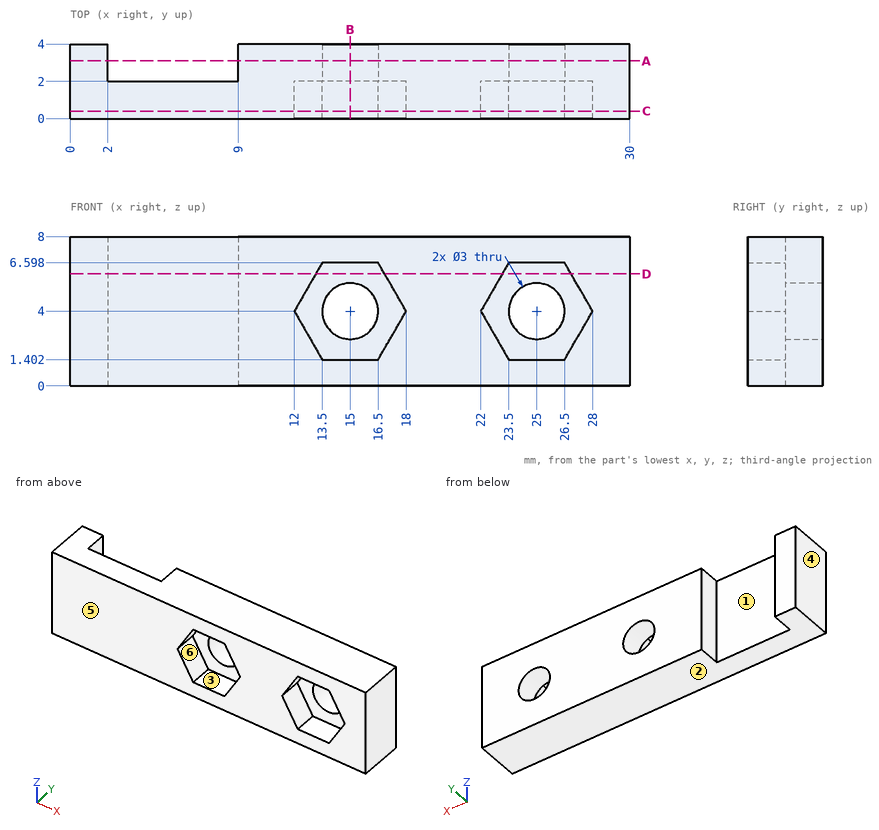
Verification items for this drawing (mm, ordinates from the low corner). A direction names the side the tool comes from. Round coordinates to 2 decimals unless told otherwise and drop trailing zeros. Loops run counter-clockwise (first coordinate to the right, second up) from the corner with the lowest first, then second, coordinate; pieces in that order, holes last. Notation, with made-up numbers: (79, 1.5) -> (107, 1.5) arc R21 ccw to (107, 17.5) -> close; hole circle Ø10 at (3, 49.25). An arc over 180 degrees is marked (long way). Write item = value, one per line. Start each with the question number.
1) Sectioned sample at C-C, the plane y = 0.4. Record the cut outline in (x, z).
2) Thickness scan on probe 1 along X at (y, z) = (3.1, 4); probe 2 along Z at (x, y) = (15.5, 1.3); probe 3 along X at (y, z) = (0.75, 2) (1 decimal). Record the ranges inside material, lowest first.
3) Sectioned sample at D-D, the plane z = 6. Record the cut outline in (x, y).
4) Gauge pin test, flat ends, axial feed: pin 1 Ø1.5 at (x, z) = (16, 5) entering from +Y; pin 2 Ø2.5 at (x, z) = (15, 3.5) entering from -Y; pin 3 Ø4 at (x, z) = (5, 2) entering from +Y. Record the tip position at first contact, or that the pin passes through.
5) Sectioned sample at A-A, the plane y = 3.1. Record the cut outline in (x, z), plus the area to 3 significant figures.
6) Release check for a two-part mould opening along X. For the marked faces 4, 5 and 6 record: released by +X, released by -X, zero draft, split by the parting line, or undercut.
7) Sectioned sample at B-B, the plane x = 15. Record the cut outline in (y, z).
8) Set-up check for the marked faces 1, 2 and 3: record each of +Z, -Z, +X, -X, +Y, -Y from which the full face is reachable in a straight line by a thin tool's end or side.
Results are:
q1.outline = (0, 0) -> (30, 0) -> (30, 8) -> (0, 8) -> close; hole (12, 4) -> (13.5, 1.4) -> (16.5, 1.4) -> (18, 4) -> (16.5, 6.6) -> (13.5, 6.6) -> close; hole (22, 4) -> (23.5, 1.4) -> (26.5, 1.4) -> (28, 4) -> (26.5, 6.6) -> (23.5, 6.6) -> close
q2.probe_1 = 0 to 2, 9 to 13.5, 16.5 to 23.5, 26.5 to 30
q2.probe_2 = 0 to 1.4, 6.6 to 8
q2.probe_3 = 0 to 13.2, 16.8 to 23.2, 26.8 to 30
q3.outline = (0, 0) -> (13.15, 0) -> (13.15, 2) -> (16.85, 2) -> (16.85, 0) -> (23.15, 0) -> (23.15, 2) -> (26.85, 2) -> (26.85, 0) -> (30, 0) -> (30, 4) -> (9, 4) -> (9, 2) -> (2, 2) -> (2, 4) -> (0, 4) -> close
q4.pin_1 = 4
q4.pin_2 = 2
q4.pin_3 = 2
q5.outline = (0, 0) -> (2, 0) -> (2, 8) -> (0, 8) -> close; (9, 0) -> (30, 0) -> (30, 8) -> (9, 8) -> close; hole circle Ø3 at (15, 4); hole circle Ø3 at (25, 4)
q5.area = 170 mm^2
q6.face_4 = released by -X
q6.face_5 = zero draft
q6.face_6 = undercut
q7.outline = (0, 0) -> (4, 0) -> (4, 2.5) -> (2, 2.5) -> (2, 1.4) -> (0, 1.4) -> close; (0, 6.6) -> (2, 6.6) -> (2, 5.5) -> (4, 5.5) -> (4, 8) -> (0, 8) -> close
q8.face_1 = +Z, -Z, +Y
q8.face_2 = -Z, +X, -X, +Y, -Y
q8.face_3 = -Y
